from build123d import *

# Parameters (mm, degrees)
SKETCH1_R           = 25.4
BOSS_EXTRUDE1_DEPTH = 170.1
SKETCH2_R           = 24.65
CUT_EXTRUDE1_DEPTH  = 174.851459585
SKETCH3_W           = 108
SKETCH3_H           = 108
BOSS_EXTRUDE2_DEPTH = 1


with BuildPart() as part:
    # Sketch1 → Boss-Extrude1 (new body)
    with BuildSketch(Plane(origin=(0, 0, 0), x_dir=(1, 0, 0), z_dir=(0, 1, 0))):
        with Locations(Location((0, 0, 0), (0, 0, 270))):
            Circle(SKETCH1_R)
    extrude(amount=BOSS_EXTRUDE1_DEPTH)

    # Sketch2 → Cut-Extrude1 (cut, through all)
    with BuildSketch(Plane(origin=(0, 170.1, 0), x_dir=(1, 0, 0), z_dir=(0, 1, 0))):
        with Locations(Location((0, 0, 0), (0, 0, 270))):
            Circle(SKETCH2_R)
    extrude(amount=-CUT_EXTRUDE1_DEPTH, mode=Mode.SUBTRACT)

    # Sketch3 → Boss-Extrude2 (add)
    with BuildSketch(Plane(origin=(0, 170.1, 0), x_dir=(1, 0, 0), z_dir=(0, 1, 0))):
        Rectangle(SKETCH3_W, SKETCH3_H)
    extrude(amount=BOSS_EXTRUDE2_DEPTH)


solid = part.part
The listing builds one solid part. Answer for the finished solid, in the listing's coordinates (mm). A direction names the side the tool comes from. Give positions to 0.01 mm unless a question says otherwise; leave off trailing zeros. Write each loop counter-clockwise with the first axis right and the second up, starting at its lowest first coordinate (ties: lowest second). Pieces come first, ordered by that corner, then holes. Notation, with made-up numbers: (-32.75, 47.25) -> (-1.75, 47.25) arc R25 ccw to (-1.75, 84.25) -> close; hole circle Ø1 at (59.25, -3.5). An arc over 180 degrees is marked (long way). Use a Markdown table: item, result.
(1) Flat-ended cylindrical pins translate along their axes: P1, Ø5, axis at x = 30, z = -5, coming from the -Y side; P2, Ø3, axis at x = 28.5, y = 30.5, coming from the -Z side; P3, Ø1.5, axis at x = -9, y = 65.5, coming from the -Z side; P4, Ø10, axis at x = -13, y = 20, coming from the +Z side. Find the tip coordinate at first contact, or state that the pin passes through.
Return value:
| item | result |
|---|---|
| P1 | y = 170.1 |
| P2 | through |
| P3 | z = -24.02 |
| P4 | z = 24.11 |
(2) For faces 4 (the flat face through (25, 0, -2)), 5 (the flat face through (0, 170.1, 0)), determine the directions among +Z, -Z, +X, -X, +Y, -Y from which every point of the face is accessible in a straight line to the end or side of a thin tool.
Return value:
| item | result |
|---|---|
| face 4 | +Z, -Z, +X, -X, -Y |
| face 5 | -Y |
(3) Find the intervals of material crossed by probe 1 along X at (y, z) = (91, 0); probe 2 along Y at (x, z) = (20, -1); probe 3 along Z at (x, y) = (4, 46), in increasing order. Write a range as from..to.
Return value:
| item | result |
|---|---|
| probe 1 | -25.4..-24.65, 24.65..25.4 |
| probe 2 | 170.1..171.1 |
| probe 3 | -25.08..-24.32, 24.32..25.08 |
(4) Section B-B, the plane z = 0 is taken. Determine the outline of the cut face in (x, y), then the cut area to 3 significant figures.
Return value:
| item | result |
|---|---|
| outline | (-54, 170.1) -> (-25.4, 170.1) -> (-25.4, 0) -> (-24.65, 0) -> (-24.65, 170.1) -> (24.65, 170.1) -> (24.65, 0) -> (25.4, 0) -> (25.4, 170.1) -> (54, 170.1) -> (54, 171.1) -> (-54, 171.1) -> close |
| area | 363 mm2 |
(5) Section A-A, the plane x = 0 is taken. Determine the outline of the cut face in (y, z), then the cut area to 3 significant figures.
Return value:
| item | result |
|---|---|
| outline | (0, -25.4) -> (170.1, -25.4) -> (170.1, -54) -> (171.1, -54) -> (171.1, 54) -> (170.1, 54) -> (170.1, 25.4) -> (0, 25.4) -> (0, 24.65) -> (170.1, 24.65) -> (170.1, -24.65) -> (0, -24.65) -> close |
| area | 363 mm2 |
(6) Section D-D, the plane x = -28 is taken. Determine the outline of the cut face in (y, z).
Return value:
| item | result |
|---|---|
| outline | (170.1, -54) -> (171.1, -54) -> (171.1, 54) -> (170.1, 54) -> close |
(7) Determine the mould class of faces 1 (the cylindrical face through (24.44, 86.24, -3.21)), 2 (the cylindrical face through (-15.456, 83.859, -20.157)), 3 (the flat face through (-1, 171.1, -1)) for opening direction Z: released by +Z, released by -Z, zero draft, split by the parting line, or undercut.
Return value:
| item | result |
|---|---|
| face 1 | undercut |
| face 2 | split by the parting line |
| face 3 | zero draft |
(8) Section C-C, the plane y = 108 is taken. Determine the outline of the cut face in (x, z).
Return value:
| item | result |
|---|---|
| outline | circle Ø50.8 at (0, 0); hole circle Ø49.3 at (0, 0) |
